```python
from build123d import *

# Parameters (mm, degrees)
F1_DEPTH = 9
F2_R     = 8


with BuildPart() as f1:
    # F0 (on Front) → F1 (new body)
    with BuildSketch(Plane.XZ):
        with BuildLine():
            ThreePointArc((-42.5, -63), (-38.106602, -73.606602), (-27.5, -78))
            Line((-27.5, -78), (27.5, -78))
            ThreePointArc((27.5, -78), (38.106602, -73.606602), (42.5, -63))
            Line((42.5, -63), (42.5, 63))
            ThreePointArc((42.5, 63), (38.106602, 73.606602), (27.5, 78))
            Line((27.5, 78), (-27.5, 78))
            ThreePointArc((-27.5, 78), (-38.106602, 73.606602), (-42.5, 63))
            Line((-42.5, 63), (-42.5, -63))
        make_face()
    extrude(amount=F1_DEPTH)

    # F2
    f2_edges = [f1.edges().sort_by_distance(p)[0] for p in [
        (-38.106602, 0, -73.606602),
        (0, 0, -78),
        (38.106602, 0, -73.606602),
        (42.5, 0, 0),
        (38.106602, 0, 73.606602),
        (0, 0, 78),
        (-38.106602, 0, 73.606602),
        (-42.5, 0, 0),
    ]]
    fillet(f2_edges, radius=F2_R)


solid = f1.part
```
Source: CAD feature listing. Evaluate the final solid. Frame: model axes, mm. Give positions to 0.01 mm unless a question says otherwise; leave off trailing zeros. Loops run counter-clockwise (first coordinate to the right, second up) from the corner with the lowest first, then second, coordinate; pieces in that order, holes last. Notation, with made-up numbers: (67.5, 67) -> (103.5, 67) arc R28 cw to (103.5, 88) -> close; hole circle Ø4 at (-37.5, 54.25). An arc over 180 degrees is marked (long way). Put each result on its own line as item: value. Start each with the question number.
1) Contact query for flat-ended pins moving along their axis: P1, Ø2, axis at x = 6, y = -2.5, coming from the -Z side; P2, Ø3, axis at y = -4.5, z = 22.5, coming from the -X side; P3, Ø1.5, axis at y = -1, z = -46.5, coming from the +X side. Output: stop coordinate, or through.
2) Material intervals for probe 1 along Z at (x, y) = (6.5, -7.5); probe 2 along X at (y, z) = (-5.5, -8); probe 3 along Z at (x, y) = (2, -1.25), sorted ascending.
3) Cut plane B-B (x = 17.5). Return loops of the section in (y, z), then the cut area to 3 significant figures.
4) Cut plane A-A (z = -14.5). Return loops of the section in (x, y), then the cut area to 3 significant figures.
5) Draft query along Y for faces 1 (the face through (-1, -9, 1)), 2 (the face through (37.99, -8.49, -73.72)), 3 (the face through (-0.385, -2.406, 75.719)). Return one class per face: released by +Y, released by -Y, zero draft, split by the parting line, or undercut.
Results are:
1. P1: stops at z = -76.61
1. P2: stops at x = -42.25
1. P3: stops at x = 39.49
2. probe 1: z = -77.98 to 77.98
2. probe 2: x = -42.1 to 42.1
2. probe 3: z = -74.29 to 74.29
3. outline: (-9, -78) -> (-8, -78) arc R8 ccw to (0, -70) -> (0, 70) arc R8 ccw to (-8, 78) -> (-9, 78) -> close
3. area: 1,380 mm2
4. outline: (-42.5, -9) -> (42.5, -9) -> (42.5, -8) arc R8 ccw to (34.5, 0) -> (-34.5, 0) arc R8 ccw to (-42.5, -8) -> close
4. area: 738 mm2
5. face 1: released by -Y
5. face 2: zero draft
5. face 3: released by +Y
